```python
from build123d import *

# Parameters (mm, degrees)
BOSS_EXTRUDE1_DEPTH     = 35
CUT_EXTRUDE1_DEPTH      = 124.917223134
CUT_EXTRUDE1_DEPTH_BACK = 124.917223134
SKETCH2_W               = 8
SKETCH2_H               = 45
CUT_EXTRUDE2_DEPTH      = 124.917223134
CUT_EXTRUDE2_DEPTH_BACK = 124.917223134
SKETCH3_R               = 15
CUT_EXTRUDE3_DEPTH      = 124.917223134
CUT_EXTRUDE3_DEPTH_BACK = 124.917223134
SKETCH4_R               = 15
SKETCH5_R               = 30
BOSS_EXTRUDE2_DEPTH     = 75


with BuildPart() as part:
    # Sketch1 → Boss-Extrude1 (new body)
    with BuildSketch(Plane.XY):
        with BuildLine():
            Line((-40, -104.548927251), (-40, 104.548927251))
            ThreePointArc((-40, 104.548927251), (0, 111.939618497), (40, 104.548927251))
            Line((40, 104.548927251), (40, -104.548927251))
            ThreePointArc((40, -104.548927251), (0, -111.939618497), (-40, -104.548927251))
        make_face()
    extrude(amount=BOSS_EXTRUDE1_DEPTH)

    # Sketch2 → Cut-Extrude1 (cut, two sides: drawn at the far end of the back side and taken through both)
    with BuildSketch(Plane(origin=(0, 0, 0), x_dir=(0, 0, -1), z_dir=(1, 0, 0)).offset(-CUT_EXTRUDE1_DEPTH_BACK)):
        with Locations((-31, 0)):
            Rectangle(SKETCH2_W, SKETCH2_H)
    extrude(amount=CUT_EXTRUDE1_DEPTH + CUT_EXTRUDE1_DEPTH_BACK, mode=Mode.SUBTRACT)

    # Sketch3 → Cut-Extrude2 (cut, two sides: drawn at the far end of the back side and taken through both)
    with BuildSketch(Plane.XY.offset(-CUT_EXTRUDE2_DEPTH_BACK)):
        with Locations((0, 74.548927251)):
            Circle(SKETCH3_R)
    extrude(amount=CUT_EXTRUDE2_DEPTH + CUT_EXTRUDE2_DEPTH_BACK, mode=Mode.SUBTRACT)

    # Sketch4 → Cut-Extrude3 (cut, two sides: drawn at the far end of the back side and taken through both)
    with BuildSketch(Plane.XY.offset(-CUT_EXTRUDE3_DEPTH_BACK)):
        with Locations((0, -75.451072749)):
            Circle(SKETCH4_R)
    extrude(amount=CUT_EXTRUDE3_DEPTH + CUT_EXTRUDE3_DEPTH_BACK, mode=Mode.SUBTRACT)

    # Sketch5 → Boss-Extrude2 (add)
    with BuildSketch(Plane(origin=(0, 0, 0), x_dir=(-1, 0, 0), z_dir=(0, 0, -1))):
        with Locations(Location((0, 0, 0), (0, 0, 180))):
            Circle(SKETCH5_R)
    extrude(amount=BOSS_EXTRUDE2_DEPTH)


solid = part.part
```
Can you work these out from the model? Positions are in its coordinate system, mm. A direction names the side the tool comes from. Coordinates: 2 decimals unless noted, no trailing zeros. Order: outer loops, then holes, each group sorted by start corner. A loop starts at its lowest first (then second) coordinate and runs counter-clockwise, first axis right, second up.
1. If we section it at A-A (x = 0): Please give me the cut outline in (y, z), then the cut area to 3 significant figures.
2. If we section it at C-C (y = 0): Please give me the cut outline in (x, z).
3. If we section it at B-B (y = -78): Please give me the cut outline in (x, z), then the cut area to 3 significant figures.
4. I need wall thicknesses on line 1 (Y direction, x = 0, z = 21); line 2 (Z direction, x = -3, y = 49); line 3 (Z direction, x = 1.5, y = 11). Which ranges of each line are inside material? Lowest first, please.
5. If we section it at D-D (x = 18.5): Please give me the cut outline in (y, z), then the cut area to 3 significant figures.
6. Thinking about a two-plate mould opening in Y: for faces 3 (the face through (1, -57, 35)), 4 (the face through (16.128, -25.296, -36.975)), 5 (the face through (-1, 0, 27)), which applies, +Y half, -Y half, draft (parallel to the pull), parting line (faces both ways), or undercut?
7. For faces 1 (the face through (-1, -22.5, 31)), 2 (the face through (-3.252, 59.906, 17.255)), which set-ups out of +Z, -Z, +X, -X, +Y, -Y let a thin tool reach every point of the face, with its end or its side?
8. I'm going to push flat-ended pins straight in: pin 1 (10 mm diameter, centred on x = 14, z = -2.5, fed in from +Y); pin 2 (2.5 mm diameter, centred on x = 8.5, z = 29, fed in from +Y); pin 3 (6 mm diameter, centred on x = -26, z = 22.5, fed in from -Y); pin 4 (4 mm diameter, centred on y = 46.5, z = -3.5, fed in from +X). Where does each tip first touch, or does it pass through?
Entries:
1. outline: (-111.94, 0) - (-90.45, 0) - (-90.45, 35) - (-111.94, 35) - close; (-60.45, 0) - (-30, 0) - (-30, -75) - (30, -75) - (30, 0) - (59.55, 0) - (59.55, 35) - (22.5, 35) - (22.5, 27) - (-22.5, 27) - (-22.5, 35) - (-60.45, 35) - close; (89.55, 0) - (111.94, 0) - (111.94, 35) - (89.55, 35) - close
1. area: 9,880 mm2
2. outline: (-40, 0) - (-30, 0) - (-30, -75) - (30, -75) - (30, 0) - (40, 0) - (40, 27) - (-40, 27) - close
3. outline: (-40, 0) - (-14.78, 0) - (-14.78, 35) - (-40, 35) - close; (14.78, 0) - (40, 0) - (40, 35) - (14.78, 35) - close
3. area: 1,770 mm2
4. line 1: y = -111.94 to -90.45, -60.45 to 59.55, 89.55 to 111.94
4. line 2: z = 0 to 35
4. line 3: z = -75 to 27
5. outline: (-110.4, 0) - (-23.62, 0) - (-23.62, -75) - (23.62, -75) - (23.62, 0) - (110.4, 0) - (110.4, 35) - (22.5, 35) - (22.5, 27) - (-22.5, 27) - (-22.5, 35) - (-110.4, 35) - close
5. area: 10,900 mm2
6. face 3: draft
6. face 4: parting line
6. face 5: undercut
7. face 1: +Z, +X, -X
7. face 2: +Z, -Z
8. pin 1: stops at y = 111.52
8. pin 2: stops at y = 111.7
8. pin 3: stops at y = -109.55
8. pin 4: passes through
